Model file for the job. Use its own axes, mm. Face numbers are marked on the shaded views. A direction names the side the tool comes from. Round coordinates to 2 decimals unless told otherwise and drop trailing zeros. Order: outer loops, then holes, each group sorted by start corner. A loop starts at its lowest first (then second) coordinate and runs counter-clockwise, first axis right, second up. Notation, with made-up numbers: M 49,52.5 L 65,52.5 A16 cw 65,77.5 Z; hole C 43,-4.75 d7. An arc over 180 degrees is marked long. Return JSON: item names as keys, results as strings. Group by question number.
Item 1: Slice it at A-A on x = 0. Write the cut outline in (y, z) (3 decimals), then the cut area to 3 significant figures.
Item 2: Slice it at B-B on z = 0. Write the cut outline in (x, y) (3 decimals).
Item 3: Which spindle directions (+Z, -Z, +X, -X, +Y, -Y) get a long thin tool onto all of the face, cutting with end or side? Do the marked faces 1 and 2. Say none if no direction does.
Item 4: Slice it at C-C on y = -8.45. Write the cut outline in (x, z) (3 decimals).
Item 5: Slice it at D-D on z = 4.5. Write the cut outline in (x, y).
Item 6: Probe line 1 along Z through (x, y) = (0, -9.2) (3 decimals); line 2 along Z through (x, y) = (0, -7.45) (3 decimals); line 3 along Y through (x, z) = (10.5, 2). List the from-to ranges inside material, lowest first.
Item 7: Pin check, flat tips, straight feed: pin 1 Ø1.5 at (y, z) = (-7.5, 0.5) entering from -X; pin 2 Ø1.5 at (x, z) = (-9.5, 4) entering from -Y; pin 3 Ø5.5 at (x, z) = (0, 0) entering from +Y. Stop position of each tip, or through.
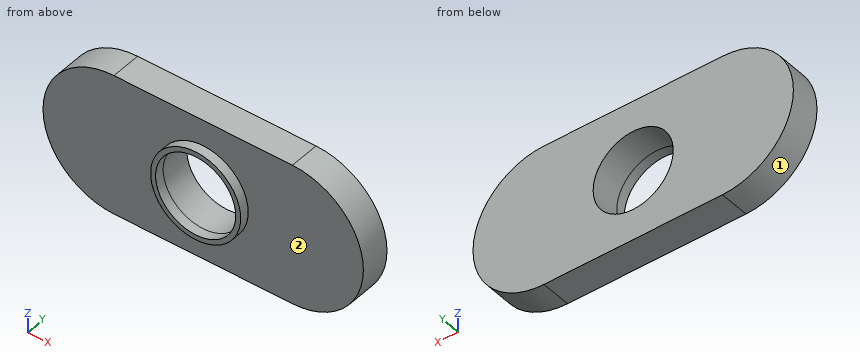
from build123d import *

# Parameters (mm, degrees)
BOSS_EXTRUDE2_START = -6.35
SKETCH8_R           = 3.175
BOSS_EXTRUDE2_DEPTH = 2.3876
SKETCH9_R           = 3.5687
SKETCH9_R_2         = 3.175
BOSS_EXTRUDE3_DEPTH = 0.762


with BuildPart() as part:
    # Sketch8 → Boss-Extrude2 (new body)
    with BuildSketch(Plane(origin=(0, 0, 0), x_dir=(1, 0, 0), z_dir=(0, 1, 0)).offset(BOSS_EXTRUDE2_START)):
        with BuildLine():
            Line((-7.0739, 5.6261), (7.0739, 5.6261))
            ThreePointArc((7.0739, 5.6261), (12.7, 0), (7.0739, -5.6261))
            Line((7.0739, -5.6261), (-7.0739, -5.6261))
            ThreePointArc((-7.0739, -5.6261), (-12.7, 0), (-7.0739, 5.6261))
        make_face()
        Circle(SKETCH8_R, mode=Mode.SUBTRACT)
    extrude(amount=-BOSS_EXTRUDE2_DEPTH)

    # Sketch9 → Boss-Extrude3 (add)
    with BuildSketch(Plane.XZ.offset(8.7376)):
        Circle(SKETCH9_R)
        Circle(SKETCH9_R_2, mode=Mode.SUBTRACT)
    extrude(amount=BOSS_EXTRUDE3_DEPTH)


solid = part.part
Output values:
{
 "1": {"outline": "M -9.5,-3.569 L -8.738,-3.569 L -8.738,-5.626 L -6.35,-5.626 L -6.35,-3.175 L -9.5,-3.175 Z; M -9.5,3.175 L -6.35,3.175 L -6.35,5.626 L -8.738,5.626 L -8.738,3.569 L -9.5,3.569 Z", "area": "12.3 mm²"},
 "2": {"outline": "M -12.7,-8.738 L -3.569,-8.738 L -3.569,-9.5 L -3.175,-9.5 L -3.175,-6.35 L -12.7,-6.35 Z; M 3.175,-9.5 L 3.569,-9.5 L 3.569,-8.738 L 12.7,-8.738 L 12.7,-6.35 L 3.175,-6.35 Z"},
 "3": {"face 1": "-X, +Y, -Y", "face 2": "-Y"},
 "4": {"outline": "M -7.074,-5.626 L 7.074,-5.626 A5.626 ccw 7.074,5.626 L -7.074,5.626 A5.626 ccw Z; hole C 0,0 d6.35"},
 "5": {"outline": "M -10.45,-8.74 L 10.45,-8.74 L 10.45,-6.35 L -10.45,-6.35 Z"},
 "6": {"line 1": "-3.569 to -3.175, 3.175 to 3.569", "line 2": "-5.626 to -3.175, 3.175 to 5.626", "line 3": "-8.74 to -6.35"},
 "7": {"pin 1": "x = -12.7", "pin 2": "y = -8.74", "pin 3": "through"}
}
